Model file for the job. Use its own axes, mm. Face numbers are marked on the shaded views. A direction names the side the tool comes from. Round coordinates to 2 decimals unless told otherwise and drop trailing zeros. Loops run counter-clockwise (first coordinate to the right, second up) from the corner with the lowest first, then second, coordinate; pieces in that order, holes last. Notation, with made-up numbers: M 80,-17.75 L 84,-17.75 A16 ccw 84,11.25 Z; hole C 37.5,-24 d8. An arc over 180 degrees is marked long. Use a Markdown table: item, result. Add a question column.
Item 1: Wall check: L1, parallel to Z at x = 0.25, y = -2; L2, parallel to Y at x = -0.5, z = 33; L3, parallel to X at y = -1, z = 8. Give the ranges that are in metal, low to high. Write a range as from..to.
Item 2: Saw through at B-B on y = 0. Write the cut outline in (x, z) (3 decimals), then the cut area to 3 significant figures.
Item 3: Tool access for the marked faces 1 and 2: list every direction of +Z, -Z, +X, -X, +Y, -Y with a clear straight run to the whole face (end or side of a thin tool).
Item 4: Saw through at D-D on y = 3.25. Write the cut outline in (x, z), then the cut area to 3 significant figures.
Item 5: Pin check, flat tips, straight feed: P1, Ø3, axis at x = -2.5, z = 25.5, coming from the +Y side; P2, Ø2, axis at y = -2.5, z = 23, coming from the -X side; P3, Ø2, axis at x = 1, z = 19.5, coming from the -Y side (3 decimals). Stop position of each tip, or through.
Item 6: Saw through at A-A on x = 3. Write the cut outline in (y, z), then the cut area to 3 significant figures.
```python
from build123d import *

# Parameters (mm, degrees)
SKETCH1_R           = 1.905
BOSS_EXTRUDE1_DEPTH = 45.72
SKETCH4_R           = 3.81
BOSS_EXTRUDE2_DEPTH = 2.54


with BuildPart() as part:
    # Sketch1 → Boss-Extrude1 (new body)
    with BuildSketch(Plane.XY):
        Circle(SKETCH1_R)
    extrude(amount=BOSS_EXTRUDE1_DEPTH)

    # Sketch4 → Boss-Extrude2 (add)
    with BuildSketch(Plane.XY.offset(45.72)):
        Circle(SKETCH4_R)
    boss_extrude2 = extrude(amount=BOSS_EXTRUDE2_DEPTH)

    # Mirror1: Boss-Extrude2 across plane
    add(boss_extrude2.mirror(Plane.XY.offset(22.86)))


solid = part.part
```
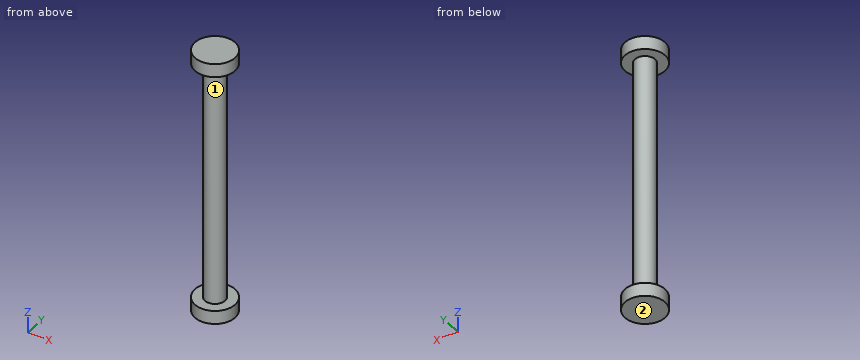
Entries:
| question | item | result |
|---|---|---|
| 1 | L1 | -2.54..0, 45.72..48.26 |
| 1 | L2 | -1.84..1.84 |
| 1 | L3 | -1.62..1.62 |
| 2 | outline | M -3.81,-2.54 L 3.81,-2.54 L 3.81,0 L 1.905,0 L 1.905,45.72 L 3.81,45.72 L 3.81,48.26 L -3.81,48.26 L -3.81,45.72 L -1.905,45.72 L -1.905,0 L -3.81,0 Z |
| 2 | area | 213 mm2 |
| 3 | face 1 | none |
| 3 | face 2 | -Z, +X, -X, +Y, -Y |
| 4 | outline | M -1.99,-2.54 L 1.99,-2.54 L 1.99,0 L -1.99,0 Z; M -1.99,45.72 L 1.99,45.72 L 1.99,48.26 L -1.99,48.26 Z |
| 4 | area | 20.2 mm2 |
| 5 | P1 | y = 1.62 |
| 5 | P2 | x = -1.17 |
| 5 | P3 | y = -1.905 |
| 6 | outline | M -2.35,-2.54 L 2.35,-2.54 L 2.35,0 L -2.35,0 Z; M -2.35,45.72 L 2.35,45.72 L 2.35,48.26 L -2.35,48.26 Z |
| 6 | area | 23.9 mm2 |
